from build123d import *

# Parameters (mm, degrees)
F0_R     = 0.5
F1_DEPTH = 17.5
F2_R     = 2.5
F3_DEPTH = 2.5
F4_SIZE  = 1
F5_R     = 2.522448
F6_DEPTH = 2.5
F7_SIZE  = 1


with BuildPart() as f1:
    # F0 (on Right) → F1 (new body, symmetric)
    with BuildSketch(Plane.YZ):
        Circle(F0_R)
    extrude(amount=F1_DEPTH, both=True)

    # F2 (on Right) → F3 (join)
    with BuildSketch(Plane.YZ):
        Circle(F2_R)
    extrude(amount=F3_DEPTH)

    # F4
    f4_edges = [f1.edges().sort_by_distance(p)[0] for p in [
        (0, -2.5, 0),
    ]]
    chamfer(f4_edges, length=F4_SIZE)

    # F5 (on Right) → F6 (join)
    with BuildSketch(Plane.YZ):
        Circle(F5_R)
    extrude(amount=-F6_DEPTH)

    # F7
    f7_edges = [f1.edges().sort_by_distance(p)[0] for p in [
        (0, -2.522448, 0),
    ]]
    chamfer(f7_edges, length=F7_SIZE)


solid = f1.part
Geometry: final body of the model. Coordinates: model frame, mm. A direction names the side the tool comes from. Coordinates: 2 decimals unless noted, no trailing zeros. Order: outer loops, then holes, each group sorted by start corner. A loop starts at its lowest first (then second) coordinate and runs counter-clockwise, first axis right, second up.
(1) First-contact query: pin 1 (1 mm diameter, centred on x = 8, z = 2, fed in from +Y); pin 2 (1.5 mm diameter, centred on y = 1, z = -1, fed in from +X); pin 3 (1.5 mm diameter, centred on x = -6.5, y = -0.5, fed in from +Z); pin 4 (1.5 mm diameter, centred on y = -0.5, z = -2, fed in from -X). Flat tips, straight axial feed; report the tip coordinate or a pass-through.
(2) Section query C-C (x = 13.5). Return the cut outline in (y, z), plus the area to 3 significant figures.
(3) Access query for faces 1 (the face through (10.105, -0.108, -0.488)), 2 (the face through (-1.74, -2.002, -1.535)), 3 (the face through (-9.895, -0.108, -0.488)). Directions: +Z, -Z, +X, -X, +Y, -Y. A direction counts if a zero-diameter tool reaches every point of the face in a straight line with its end or side. Return the directions, or none.
(4) Material intervals for probe 1 along X at (y, z) = (-0.5, -0.25); probe 2 along X at (y, z) = (-0.05, 1.6); probe 3 along X at (y, z) = (-1.3, 1.65), sorted ascending.
Solution:
1. pin 1: passes through
1. pin 2: stops at x = 2.5
1. pin 3: stops at z = 0.5
1. pin 4: stops at x = -2.5
2. outline: circle Ø1 at (0, 0)
2. area: 0.785 mm2
3. face 1: +X
3. face 2: +X, -X
3. face 3: -X
4. probe 1: x = -2.5 to 2.5
4. probe 2: x = -2.5 to -0.08, 0.1 to 2.5
4. probe 3: x = -2.5 to -0.58, 0.6 to 2.5
